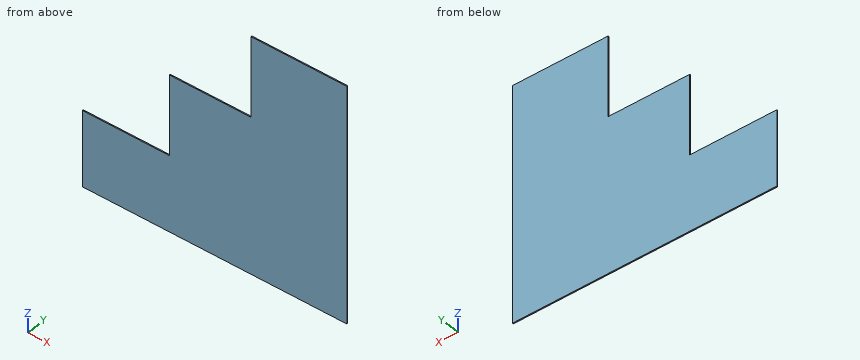
from build123d import *

# Parameters (mm, degrees)
F0_W     = 375
F0_H     = 355
F0_W_2   = 440
F0_H_2   = 20
F1_DEPTH = 5


with BuildPart() as f1:
    # F0 (on Front) → F1 (new body)
    with BuildSketch(Plane.XZ):
        Polygon((-815, 0), (-1215, 0), (-1215, -355), (0, -355), (0, 0), (-440, 0), align=None)
        with Locations((-627.5, 197.5)):
            Rectangle(F0_W, F0_H)
        with Locations((-220, 197.5)):
            Rectangle(F0_W_2, F0_H)
        with Locations((-220, 572.5)):
            Rectangle(F0_W_2, F0_H)
        with Locations((-220, 385)):
            Rectangle(F0_W_2, F0_H_2)
        with Locations((-220, 10)):
            Rectangle(F0_W_2, F0_H_2)
        with Locations((-627.5, 10)):
            Rectangle(F0_W, F0_H_2)
    extrude(amount=F1_DEPTH)


solid = f1.part
Design review of the part built by this model. Coordinates are the model's own, in mm. Give positions to 0.01 mm unless a question says otherwise; leave off trailing zeros. Write each loop counter-clockwise with the first axis right and the second up, starting at its lowest first coordinate (ties: lowest second). Pieces come first, ordered by that corner, then holes. Notation, with made-up numbers: M -20,11 L 19,11 A28 ccw 19,49 Z; hole C 75.25,25 d6. An arc over 180 degrees is marked long. Answer as a JSON object with one key per item and string values. Group by question number.
1) We need section C-C (z = 434.5). Give the boundary of the cut face in (x, y), and give its area (3 significant figures).
2) We need section A-A (y = -0.8). Give the boundary of the cut face in (x, z), and give its area (3 significant figures).
3) We need section B-B (x = -1122). Give the boundary of the cut face in (y, z), and give its area (4 significant figures).
4) For line 1 along X through (y, z) = (-1.2, 695); line 2 along X through (y, z) = (-3.65, 143.5); line 3 along Z through (x, y) = (-742.5, -3.8), list the stretches that pass through material, from the lowest coordinate up.
5) Clearance check with flat-ended pins moving along their axes: pin 1 Ø8 at (x, z) = (-1056, -214.5) entering from +Y; pin 2 Ø2.5 at (y, z) = (-3, 126.5) entering from -X; pin 3 Ø2.5 at (x, y) = (-560, -3.5) entering from +Z; pin 4 Ø2.5 at (x, y) = (-1017, -1.5) entering from +Z. State where each tip first meets the part, or that it passes through.
Answer key:
{
 "1": {"outline": "M -440,-5 L 0,-5 L 0,0 L -440,0 Z", "area": "2,200 mm²"},
 "2": {"outline": "M -1215,-355 L 0,-355 L 0,750 L -440,750 L -440,375 L -815,375 L -815,0 L -1215,0 Z", "area": "902,000 mm²"},
 "3": {"outline": "M -5,-355 L 0,-355 L 0,0 L -5,0 Z", "area": "1,775 mm²"},
 "4": {"line 1": "x = -440 to 0", "line 2": "x = -815 to 0", "line 3": "z = -355 to 375"},
 "5": {"pin 1": "stops at y = 0", "pin 2": "stops at x = -815", "pin 3": "stops at z = 375", "pin 4": "stops at z = 0"}
}
